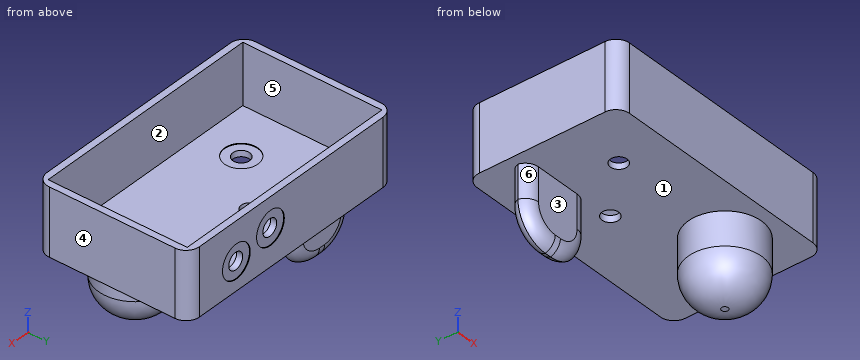
from build123d import *

# Parameters (mm, degrees)
F0_W           = 94.2332278937
F0_H           = 57.9777825624
F1_DEPTH       = 25.4
F2_T           = -2.54
F3_R           = 5.08
F5_D           = 6.35
F7_D           = 6.35
F7_DEPTH       = 12.7
F7_CBORE_D     = 12.7
F7_CBORE_DEPTH = 0.254
F7_TIP         = 1.9077324654
F9_D           = 6.35
F9_DEPTH       = 12.7
F9_CBORE_D     = 12.7
F9_CBORE_DEPTH = 0.254
F9_TIP         = 1.9077324654
F10_R          = 13.9169366501
F11_DEPTH      = 25.4
F12_R          = 12.7
F13_W          = 27.7714207768
F13_H          = 7.534484379
F14_DEPTH      = 25.4
F15_R          = 12.7
F16_T1_DEPTH   = 12.7
F16_T3_DEPTH   = 2.3714207768
F16_T6_ANGLE   = 90
F16_T8_ANGLE   = 90
F16_T10_ANGLE  = 90
F16_T12_ANGLE  = 90


# Not quite as in the source:
# - a fillet or chamfer that OpenCascade refuses, or shapes differently, is made with other operations: its cross-section is extruded or revolved along the edge and cut away or added


with BuildPart() as f1:
    # F0 (on Top) → F1 (new body)
    with BuildSketch(Plane.XY):
        with Locations((-38.147569634, 3.4275231883)):
            Rectangle(F0_W, F0_H)
    extrude(amount=F1_DEPTH)

    # F2
    f2_openings = [f1.faces().sort_by_distance(p)[0] for p in [
        (-38.14757, 3.427523, 25.4),
    ]]
    offset(amount=F2_T, openings=f2_openings)

    # F3
    f3_edges = [f1.edges().sort_by_distance(p)[0] for p in [
        (-85.264184, -25.561368, 12.7),
        (8.969044, -25.561368, 12.7),
        (8.969044, 32.416414, 12.7),
        (-85.264184, 32.416414, 12.7),
    ]]
    fillet(f3_edges, radius=F3_R)

    # F5 (through all)
    with Locations(Plane.XY.offset(2.54)):
        with Locations((-44.2425459623, 11.5331579)):
            Hole(F5_D / 2)

    # F7
    with Locations(Plane.XY.offset(2.54)):
        with Locations((-63.0617812276, -7.2897328064)):
            CounterBoreHole(F7_D / 2, F7_CBORE_D / 2, F7_CBORE_DEPTH, depth=F7_DEPTH)
            with Locations((0, 0, -(F7_DEPTH + F7_TIP / 2))):  # 118° drill point
                Cone(0, F7_D / 2, F7_TIP, mode=Mode.SUBTRACT)

    # F9
    with Locations(Plane(origin=(0, 32.4164144695, 0), x_dir=(-1, 0, 0), z_dir=(0, 1, 0))):
        with Locations((13.0262067541, 10.6704961509), (28.6341179162, 14.0921706334)):
            CounterBoreHole(F9_D / 2, F9_CBORE_D / 2, F9_CBORE_DEPTH, depth=F9_DEPTH)
            with Locations((0, 0, -(F9_DEPTH + F9_TIP / 2))):  # 118° drill point
                Cone(0, F9_D / 2, F9_TIP, mode=Mode.SUBTRACT)

    # F10 (on face) → F11 (join)
    with BuildSketch(Plane(origin=(0, 0, 0), x_dir=(1, 0, 0), z_dir=(0, 0, -1))):
        with Locations((-14.1745125875, 7.0280302316)):
            Circle(F10_R)
    extrude(amount=F11_DEPTH)

    # F12
    f12_edges = [f1.edges().sort_by_distance(p)[0] for p in [
        (-28.091449, -7.02803, -25.4),
    ]]
    fillet(f12_edges, radius=F12_R)

    # F13 (on face) → F14 (join)
    with BuildSketch(Plane(origin=(0, 0, 0), x_dir=(1, 0, 0), z_dir=(0, 0, -1))):
        with Locations((-67.7874796093, -15.7441017218)):
            Rectangle(F13_W, F13_H)
    extrude(amount=F14_DEPTH)

    # F15
    f15_edges = [f1.edges().sort_by_distance(p)[0] for p in [
        (-53.901769, 15.744102, -25.4),
        (-81.67319, 15.744102, -25.4),
    ]]
    fillet(f15_edges, radius=F15_R)

    # F16: fillet of radius 5.08 on 2 edges, made by hand

    # F16_s2 → F16_t1 (cut)
    with BuildSketch(Plane.XY.offset(-12.7)):
        with BuildLine():
            ThreePointArc((-58.9817692208, 19.5113439113), (-55.3896667724, 18.0234463597), (-53.9017692208, 14.4313439113))
            Line((-53.9017692208, 14.4313439113), (-53.9017692208, 19.5113439113))
            Line((-53.9017692208, 19.5113439113), (-58.9817692208, 19.5113439113))
        make_face()
        with BuildLine():
            ThreePointArc((-81.6731899977, 14.4313439113), (-80.1852924461, 18.0234463597), (-76.5931899977, 19.5113439113))
            Line((-76.5931899977, 19.5113439113), (-81.6731899977, 19.5113439113))
            Line((-81.6731899977, 19.5113439113), (-81.6731899977, 14.4313439113))
        make_face()
        with BuildLine():
            ThreePointArc((-81.6731899977, 17.0568595323), (-80.1852924461, 13.4647570839), (-76.5931899977, 11.9768595323))
            Line((-76.5931899977, 11.9768595323), (-81.6731899977, 11.9768595323))
            Line((-81.6731899977, 11.9768595323), (-81.6731899977, 17.0568595323))
        make_face()
        with BuildLine():
            ThreePointArc((-58.9817692208, 11.9768595323), (-55.3896667724, 13.4647570839), (-53.9017692208, 17.0568595323))
            Line((-53.9017692208, 17.0568595323), (-53.9017692208, 11.9768595323))
            Line((-53.9017692208, 11.9768595323), (-58.9817692208, 11.9768595323))
        make_face()
    extrude(amount=F16_T1_DEPTH, mode=Mode.SUBTRACT)

    # F16_s4 → F16_t3 (cut)
    with BuildSketch(Plane.YZ.offset(-68.9731899977)):
        with BuildLine():
            ThreePointArc((19.5113439113, -20.32), (18.0234463597, -23.9121024484), (14.4313439113, -25.4))
            Line((14.4313439113, -25.4), (19.5113439113, -25.4))
            Line((19.5113439113, -25.4), (19.5113439113, -20.32))
        make_face()
        with BuildLine():
            ThreePointArc((11.9768595323, -20.32), (13.4647570839, -23.9121024484), (17.0568595323, -25.4))
            Line((17.0568595323, -25.4), (11.9768595323, -25.4))
            Line((11.9768595323, -25.4), (11.9768595323, -20.32))
        make_face()
    extrude(amount=F16_T3_DEPTH, mode=Mode.SUBTRACT)

    # F16_s5 → F16_t6 (revolve, cut)
    with BuildSketch(Plane.XY.offset(-12.7)):
        with BuildLine():
            ThreePointArc((-76.5931899977, 11.9768595323), (-80.1852924461, 13.4647570839), (-81.6731899977, 17.0568595323))
            Line((-81.6731899977, 17.0568595323), (-81.6731899977, 11.9768595323))
            Line((-81.6731899977, 11.9768595323), (-76.5931899977, 11.9768595323))
        make_face()
    revolve(axis=Axis((-68.9731899977, 11.9768595323, -12.7), (0, -1, 0)), revolution_arc=F16_T6_ANGLE, mode=Mode.SUBTRACT)

    # F16_s7 → F16_t8 (revolve, cut)
    with BuildSketch(Plane.XY.offset(-12.7)):
        with BuildLine():
            ThreePointArc((-58.9817692208, 19.5113439113), (-55.3896667724, 18.0234463597), (-53.9017692208, 14.4313439113))
            Line((-53.9017692208, 14.4313439113), (-53.9017692208, 19.5113439113))
            Line((-53.9017692208, 19.5113439113), (-58.9817692208, 19.5113439113))
        make_face()
    revolve(axis=Axis((-66.6017692208, 19.5113439113, -12.7), (0, 1, 0)), revolution_arc=F16_T8_ANGLE, mode=Mode.SUBTRACT)

    # F16_s9 → F16_t10 (revolve, cut)
    with BuildSketch(Plane.XY.offset(-12.7)):
        with BuildLine():
            ThreePointArc((-81.6731899977, 14.4313439113), (-80.1852924461, 18.0234463597), (-76.5931899977, 19.5113439113))
            Line((-76.5931899977, 19.5113439113), (-81.6731899977, 19.5113439113))
            Line((-81.6731899977, 19.5113439113), (-81.6731899977, 14.4313439113))
        make_face()
    revolve(axis=Axis((-68.9731899977, 19.5113439113, -12.7), (0, -1, 0)), revolution_arc=F16_T10_ANGLE, mode=Mode.SUBTRACT)

    # F16_s11 → F16_t12 (revolve, cut)
    with BuildSketch(Plane.XY.offset(-12.7)):
        with BuildLine():
            ThreePointArc((-58.9817692208, 11.9768595323), (-55.3896667724, 13.4647570839), (-53.9017692208, 17.0568595323))
            Line((-53.9017692208, 17.0568595323), (-53.9017692208, 11.9768595323))
            Line((-53.9017692208, 11.9768595323), (-58.9817692208, 11.9768595323))
        make_face()
    revolve(axis=Axis((-66.6017692208, 11.9768595323, -12.7), (0, 1, 0)), revolution_arc=F16_T12_ANGLE, mode=Mode.SUBTRACT)


solid = f1.part
The listing builds one solid part. Answer for the finished solid, in the listing's coordinates (mm). Face numbers are marked on the shaded views. A direction names the side the tool comes from. Give positions to 0.01 mm unless a question says otherwise; leave off trailing zeros. Write each loop counter-clockwise with the first axis right and the second up, starting at its lowest first coordinate (ties: lowest second). Pieces come first, ordered by that corner, then holes.
1) Section B-B (z = -2.5) is taken. Write down the section's boundary in (x, y).
2) Given P1, Ø8, axis at x = -23.5, y = 15.5, coming from the -Z side; P2, Ø9, axis at x = -66.5, z = -14, coming from the +Y side; P3, Ø4, axis at x = -28, z = 13.5, coming from the +Y side; P4, Ø12, axis at x = -44, z = -9, coming from the -Y side, each flat-ended and moving along its own axis, determine where each tip first touches the part or whether it passes through.
3) Section D-D (z = 22) is taken. Write down the section's boundary in (x, y).
4) Find the intervals of material crossed by L1, parallel to Y at x = -75.5, z = 13; L2, parallel to X at y = 27.5, z = 13; L3, parallel to Z at x = -8, y = 26, in increasing order.
5) For a pull along X with two mould halves and no side action, classify the marked faces 4, 5 and 6 as pulls with the +X half, pulls with the -X half, needs draft (parallel to the pull), parting line crosses it, or undercut.
6) A tool of negligible diameter and unlimited length cuts with its end or side. For the marked faces 1, 2 and 3, from which of +Z, -Z, +X, -X, +Y, -Y can it reach the whole face along a straight path? Write none if from no direction.
7) Section C-C (y = 21) is taken. Write down the section's boundary in (x, z), and give its area (3 significant figures).
8) Section A-A (x = -40) is taken. Write down the section's boundary in (y, z).
Response:
1. outline: (-81.5, 15.74) arc R5.08 ccw to (-76.59, 11.98) - (-58.98, 11.98) arc R5.08 ccw to (-54.07, 15.74) arc R5.08 ccw to (-58.98, 19.51) - (-76.59, 19.51) arc R5.08 ccw to start; circle Ø27.83 at (-14.17, -7.03)
2. P1: stops at z = 0
2. P2: stops at y = 19.51
2. P3: stops at y = -23.02
2. P4: passes through
3. outline: (-85.26, -20.48) arc R5.08 ccw to (-80.18, -25.56) - (3.89, -25.56) arc R5.08 ccw to (8.97, -20.48) - (8.97, 27.34) arc R5.08 ccw to (3.89, 32.42) - (-80.18, 32.42) arc R5.08 ccw to (-85.26, 27.34) - close; hole (-82.72, -23.02) - (6.43, -23.02) - (6.43, 29.88) - (-82.72, 29.88) - close
4. L1: y = -25.56 to -23.02, 29.88 to 32.42
4. L2: x = -85.26 to -82.72, 6.43 to 8.97
4. L3: z = 0 to 2.54
5. face 4: pulls with the +X half
5. face 5: undercut
5. face 6: pulls with the -X half
6. face 1: -Z
6. face 2: +Z
6. face 3: -Z, +X, -X, -Y
7. outline: (-85.26, 0) - (8.97, 0) - (8.97, 25.4) - (6.43, 25.4) - (6.43, 2.54) - (-82.72, 2.54) - (-82.72, 25.4) - (-85.26, 25.4) - close
7. area: 355 mm2
8. outline: (-25.56, 0) - (32.42, 0) - (32.42, 25.4) - (29.88, 25.4) - (29.88, 2.54) - (-23.02, 2.54) - (-23.02, 25.4) - (-25.56, 25.4) - close
